Autodesk Inventor part; units mm, degrees
ref_plane "YZ Plane" through (0, 0, 0) normal (1, 0, 0) x (0, 1, 0)
ref_plane "XZ Plane" through (0, 0, 0) normal (0, 1, 0) x (-1, 0, 0)
ref_plane "XY Plane" through (0, 0, 0) normal (0, 0, 1) x (1, 0, 0)
sketch "Sketch1" plane through (0, 0, 0) normal (0, 0, 1) x (1, 0, 0)
  line L0 (0, 0) -> (120, 0)
  line L1 (120, 0) -> (120, 30)
  line L2 (120, 30) -> (0, 30)
  line L3 (0, 30) -> (0, 0)
  dimension "width" = 120
  dimension "d1" = 30
extrude "Extrusion1" add sketch "Sketch1" along normal blind 8
hole "Hole1" at (15, 8, 8) direction (0, 0, -1) diameter 6.5 end through all countersink diameter 10 countersink angle 90
hole "Hole2" at (105, 8, 8) direction (0, 0, -1) diameter 6.5 end through all countersink diameter 10 countersink angle 90
hole "Hole3" at (60, 18, 0) direction (0, 0, 1) diameter 16 depth 5
hole "Hole4" at (60, 18, 5) direction (0, 0, 1) diameter 5.5 end through all
hole "Hole5" at (5, 24, 8) direction (0, 0, -1) diameter 4.134 end through all
hole "Hole6" at (115, 24, 8) direction (0, 0, -1) diameter 4.134 end through all
pattern_linear "Rectangular Pattern1" count 2 spacing 32 along (1, 0, 0) of "Hole5"
pattern_linear "Rectangular Pattern2" count 2 spacing 32 along (-1, 0, 0) of "Hole6"
equation "\"d22\" = 0.5 * width"
properties part number "alu top plate"
Source: CAD feature listing. Evaluate the final solid. Frame: model axes, mm. A direction names the side the tool comes from. Coordinates: 2 decimals unless noted, no trailing zeros. Loops run counter-clockwise (first coordinate to the right, second up) from the corner with the lowest first, then second, coordinate; pieces in that order, holes last. Notation, with made-up numbers: (8.25, 49.5) - (43.25, 49.5) arc R25 cw to (43.25, 84.5) - close; hole circle Ø5 at (2, 20). An arc over 180 degrees is marked (long way). Return JSON: item names as keys, results as strings.
Q1. Section C-C, the plane z = 1.75. Return loops of the section in (x, y), plus the area to 3 significant figures.
Results:
{"outline": "(0, 0) - (120, 0) - (120, 30) - (0, 30) - close; hole circle Ø4.13 at (5, 24); hole circle Ø6.5 at (15, 8); hole circle Ø4.13 at (37, 24); hole circle Ø16 at (60, 18); hole circle Ø4.13 at (83, 24); hole circle Ø6.5 at (105, 8); hole circle Ø4.13 at (115, 24)", "area": "3,280 mm2"}
Q2. Contact query for flat-ended pins moving along their axis: P1, Ø6.5, axis at x = 83, y = 24, coming from the -Z side; P2, Ø1.5, axis at x = 66, y = 14.5, coming from the -Z side; P3, Ø3.5, axis at x = 5, y = 24, coming from the +Z side. Output: stop coordinate, or through.
Results:
{"P1": "z = 0", "P2": "z = 5", "P3": "through"}
Q3. Access query for faces 1 (the cylindrical face through (52.068, 16.959, 2.535)), 2 (the cylindrical face through (4.38, 22.03, 3.94)). Directions: +Z, -Z, +X, -X, +Y, -Y. A direction counts if a zero-diameter tool reaches every point of the face in a straight line with its end or side. Return the directions, or none.
Results:
{"face 1": "-Z", "face 2": "+Z, -Z"}
Q4. Section A-A, the plane x = 60. Return loops of the section in (y, z).
Results:
{"outline": "(0, 0) - (10, 0) - (10, 5) - (15.25, 5) - (15.25, 8) - (0, 8) - close; (20.75, 5) - (26, 5) - (26, 0) - (30, 0) - (30, 8) - (20.75, 8) - close"}
Q5. Section B-B, the plane y = 8. Return loops of the section in (x, z), plus the area to 3 significant figures.
Results:
{"outline": "(0, 0) - (11.75, 0) - (11.75, 6.25) - (10, 8) - (0, 8) - close; (18.25, 0) - (101.75, 0) - (101.75, 6.25) - (100, 8) - (20, 8) - (18.25, 6.25) - close; (108.25, 0) - (120, 0) - (120, 8) - (110, 8) - (108.25, 6.25) - close", "area": "850 mm2"}
Q6. Mould query, pull axis X, two halves, no side actions, for faces 3 (the flat face through (59, 9, 0)), 4 (the conical face through (102.96, 10.67, 6.36)), 5 (the flat face through (0, 15, 4)), 6 (the flat face through (120, 15, 4)). Classes: released by +X, released by -X, zero draft, split by the parting line, or undercut.
Results:
{"face 3": "zero draft", "face 4": "undercut", "face 5": "released by -X", "face 6": "released by +X"}
Q7. Section D-D, the plane y = 24. Return loops of the section in (x, z), plus the area to 3 significant figures.
Results:
{"outline": "(0, 0) - (2.93, 0) - (2.93, 8) - (0, 8) - close; (7.07, 0) - (34.93, 0) - (34.93, 8) - (7.07, 8) - close; (39.07, 0) - (54.71, 0) - (54.71, 5) - (65.29, 5) - (65.29, 0) - (80.93, 0) - (80.93, 8) - (39.07, 8) - close; (85.07, 0) - (112.93, 0) - (112.93, 8) - (85.07, 8) - close; (117.07, 0) - (120, 0) - (120, 8) - (117.07, 8) - close", "area": "775 mm2"}
Q8. Material intervals for line 1 along X through (y, z) = (8, 1.5); line 2 along Y through (x, z) = (60, 6.4); line 3 along X through (y, z) = (5.5, 2.75), sorted ascending.
Results:
{"line 1": "0 to 11.75, 18.25 to 101.75, 108.25 to 120", "line 2": "0 to 15.25, 20.75 to 30", "line 3": "0 to 12.92, 17.08 to 102.92, 107.08 to 120"}
